from build123d import *

# Parameters (mm, degrees)
BOSS_EXTRUDE1_DEPTH      = 8.89
BOSS_EXTRUDE1_DEPTH_BACK = 8.89
SKETCH2_R                = 7.62
BOSS_EXTRUDE3_DEPTH      = 1.3716
SKETCH4_R                = 5.88645
BOSS_EXTRUDE4_DEPTH      = 1.016
SKETCH5_R                = 6.2865
BOSS_EXTRUDE5_DEPTH      = 1.3208
SKETCH6_R                = 2.9845
CUT_EXTRUDE2_DEPTH       = 25.039137559


with BuildPart() as part:
    # Sketch1 → Boss-Extrude1 (new, two sides: drawn at the far end of the back side and taken through both)
    with BuildSketch(Plane.XY.offset(-BOSS_EXTRUDE1_DEPTH_BACK)):
        Polygon((3.763810109, 6.292620026), (-3.567663745, 6.405865183), (-7.331473854, 0.113245156), (-3.763810109, -6.292620026), (3.567663745, -6.405865183), (7.331473854, -0.113245156), align=None)
    extrude(amount=BOSS_EXTRUDE1_DEPTH + BOSS_EXTRUDE1_DEPTH_BACK)

    # Sketch2 → Boss-Extrude3 (add)
    with BuildSketch(Plane.XY.offset(8.89)):
        Circle(SKETCH2_R)
    extrude(amount=BOSS_EXTRUDE3_DEPTH)

    # Sketch4 → Boss-Extrude4 (add)
    with BuildSketch(Plane(origin=(0, 0, -8.89), x_dir=(-1, 0, 0), z_dir=(0, 0, -1))):
        with Locations(Location((0, 0, 0), (0, 0, 180))):
            Circle(SKETCH4_R)
    extrude(amount=BOSS_EXTRUDE4_DEPTH)

    # Sketch5 → Boss-Extrude5 (add)
    with BuildSketch(Plane(origin=(0, 0, -9.906), x_dir=(-1, 0, 0), z_dir=(0, 0, -1))):
        Circle(SKETCH5_R)
    extrude(amount=BOSS_EXTRUDE5_DEPTH)

    # Sketch6 → Cut-Extrude2 (cut, through all)
    with BuildSketch(Plane(origin=(0, 0, -11.2268), x_dir=(-1, 0, 0), z_dir=(0, 0, -1))):
        Circle(SKETCH6_R)
    extrude(amount=-CUT_EXTRUDE2_DEPTH, mode=Mode.SUBTRACT)


solid = part.part
Geometry check sheet. Reference: the model listing, model coordinates, mm. A direction names the side the tool comes from. Round coordinates to 2 decimals unless told otherwise and drop trailing zeros. Write each loop counter-clockwise with the first axis right and the second up, starting at its lowest first coordinate (ties: lowest second). Pieces come first, ordered by that corner, then holes.
Item 1: Section check D-D (y = -4). Record the boundary of the cut face in (x, z).
Determined:
outline: (-6.49, 8.89) - (-5.04, 8.89) - (-5.04, -8.89) - (-4.32, -8.89) - (-4.32, -9.91) - (-4.85, -9.91) - (-4.85, -11.23) - (4.85, -11.23) - (4.85, -9.91) - (4.32, -9.91) - (4.32, -8.89) - (5.01, -8.89) - (5.01, 8.89) - (6.49, 8.89) - (6.49, 10.26) - (-6.49, 10.26) - close
Item 2: Go/stop test with flat-tipped pins: pin 1 Ø4 at (y, z) = (-1, 7.5) entering from +X; pin 2 Ø5 at (x, z) = (5.5, -6) entering from +Y; pin 3 Ø1.5 at (x, z) = (-5, 4.5) entering from +Y. Record where each tip stops, or that it passes through.
Determined:
pin 1: stops at x = 7.62
pin 2: stops at y = 6.3
pin 3: stops at y = 5.27
Item 3: Material ranges on line 1 along Y through (x, z) = (3.5, -5.5); line 2 along Z through (x, y) = (-3, -6.5); line 3 along X through (y, z) = (-0.5, -6.5), recorded low to high.
Determined:
line 1: y = -6.4 to 6.3
line 2: z = 8.89 to 10.26
line 3: x = -6.99 to -2.94, 2.94 to 7.1
Item 4: Mould release check, pull along Z, two halves, no side actions. Record for faces 1 (the face through (2, 6, -8.89)), 2 (the face through (3.3, 0.1, 10.262)), 3 (the face through (0.647, -2.914, -0.633)): +Z half, -Z half, draft (parallel to the pull), parting line (faces both ways), or undercut.
Determined:
face 1: undercut
face 2: +Z half
face 3: draft
Item 5: Section check C-C (y = 5). Record the boundary of the cut face in (x, z).
Determined:
outline: (-5.75, 8.89) - (-4.41, 8.89) - (-4.41, -8.89) - (-3.11, -8.89) - (-3.11, -9.91) - (-3.81, -9.91) - (-3.81, -11.23) - (3.81, -11.23) - (3.81, -9.91) - (3.11, -9.91) - (3.11, -8.89) - (4.48, -8.89) - (4.48, 8.89) - (5.75, 8.89) - (5.75, 10.26) - (-5.75, 10.26) - close
Item 6: Access from +Z, -Z, +X, -X, +Y, -Y to the whole of each face (thin tool, end or side, straight path). Record for faces 4 (the face through (-5.88, -0.26, -9.39)), 5 (the face through (5.573, 3.045, -0.124)), 6 (the face through (5.423, -3.304, -0.124)), 7 (the face through (-5.573, -3.045, -0.124)), 8 (the face through (-6.24, -2.22, 8.89)).
Determined:
face 4: none
face 5: -Z, +X, +Y
face 6: -Z, +X, -Y
face 7: -Z, -X, -Y
face 8: -Z
Item 7: Section check B-B (x = 0). Record the boundary of the cut face in (y, z), plus the area to 3 significant figures.
Determined:
outline: (-7.62, 8.89) - (-6.35, 8.89) - (-6.35, -8.89) - (-5.89, -8.89) - (-5.89, -9.91) - (-6.29, -9.91) - (-6.29, -11.23) - (-2.98, -11.23) - (-2.98, 10.26) - (-7.62, 10.26) - close; (2.98, -11.23) - (6.29, -11.23) - (6.29, -9.91) - (5.89, -9.91) - (5.89, -8.89) - (6.35, -8.89) - (6.35, 8.89) - (7.62, 8.89) - (7.62, 10.26) - (2.98, 10.26) - close
area: 147 mm2
Item 8: Section check A-A (z = -6.25). Record the boundary of the cut face in (x, y), plus the area to 3 significant figures.
Determined:
outline: (-7.33, 0.11) - (-3.76, -6.29) - (3.57, -6.41) - (7.33, -0.11) - (3.76, 6.29) - (-3.57, 6.41) - close; hole circle Ø5.97 at (0, 0)
area: 112 mm2
